Input: part model. Units: mm. Frame: model coordinates. Face numbers are marked on the shaded views. A direction names the side the tool comes from. Coordinates: 2 decimals unless noted, no trailing zeros. Order: outer loops, then holes, each group sorted by start corner. A loop starts at its lowest first (then second) coordinate and runs counter-clockwise, first axis right, second up.
Autodesk Inventor part; units mm, degrees
ref_plane "YZ Plane" through (0, 0, 0) normal (1, 0, 0) x (0, 1, 0)
ref_plane "XZ Plane" through (0, 0, 0) normal (0, 1, 0) x (-1, 0, 0)
ref_plane "XY Plane" through (0, 0, 0) normal (0, 0, 1) x (1, 0, 0)
sketch "草圖1" plane through (0, 0, 0) normal (0, 0, 1) x (1, 0, 0)
  line L0 (0, 0) -> (50, 0)
  line L1 (50, 10) -> (10, 10)
  line L2 (10, 10) -> (10, 40)
  line L3 (10, 40) -> (30, 40)
  line L4 (30, 40) -> (30, 50)
  line L5 (30, 50) -> (0, 50)
  line L6 (0, 50) -> (0, 0)
  line L7 (50, 10) -> (50, 0)
  dimension "d0" = 50
  dimension "d1" = 10
  dimension "d2" = 30
  dimension "d3" = 30
  dimension "d4" = 10
  dimension "d5" = 50
extrude "擠出1" add sketch "草圖1" along normal mid plane 40
fillet "圓角1" radius 20 2 edges at (50, 5, 20) (50, 5, -20)
fillet "圓角2" radius 20 1 edges at (0, 0, 0)
fillet "圓角3" radius 10 1 edges at (10, 10, 0)
fillet "圓角4" radius 10 2 edges at (30, 45, 20) (30, 45, -20)
sketch "草圖2" plane through (30, 10, 0) normal (0, 1, 0) x (1, 0, 0)
  arc A0 (0, -20) -> (0, 20) centre (0, 0) ccw
  point P0 (-30, 0)
hole "孔1" at (30, 10, 0) direction (0, -1, 0) diameter 20 end through all
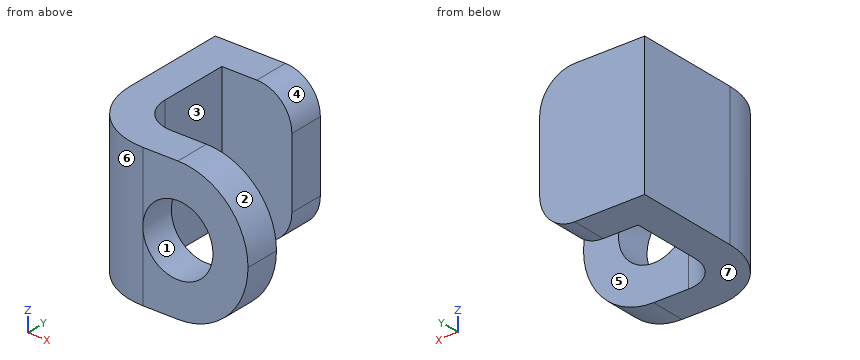
Item 1: Pin query (flat end, axial travel): pin 1 Ø16 at (y, z) = (31, -2) entering from +X; pin 2 Ø6 at (y, z) = (9.5, -3.5) entering from +X; pin 3 Ø10 at (y, z) = (43, 12.5) entering from +X; pin 4 Ø12 at (x, y) = (34.5, 33.5) entering from +Z. Return the tip coordinate at first contact, or that it passes through.
Response values:
pin 1: stops at x = 10
pin 2: stops at x = 49.99
pin 3: stops at x = 30
pin 4: passes through
Item 2: Cut plane B-B on x = 37. Return loops of the section in (y, z), then the cut area to 3 significant figures.
Response values:
outline: (0, -18.74) - (10, -18.74) - (10, -7.14) - (0, -7.14) - close; (0, 7.14) - (10, 7.14) - (10, 18.74) - (0, 18.74) - close
area: 232 mm2
Item 3: Draft query along Y for the marked faces 5, 6 and 7. Return one class per face: pulls with the +Y half, pulls with the -Y half, needs draft (parallel to the pull), parting line crosses it, or undercut.
Response values:
face 5: undercut
face 6: pulls with the -Y half
face 7: needs draft
Item 4: Ray query, probe 1 along Z at (x, y) = (30, 2); probe 2 along Y at (x, z) = (20, 16.5); probe 3 along Y at (x, z) = (41.5, 2). Return the intervals inside material, ascending.
Response values:
probe 1: z = -20 to -10, 10 to 20
probe 2: y = 0 to 10, 40 to 50
probe 3: y = 0 to 10
Item 5: Access query for the marked faces 1, 2, 3 and 4. Directions: +Z, -Z, +X, -X, +Y, -Y. A direction counts if a zero-diameter tool reaches every point of the face in a straight line with its end or side. Return the directions, or none.
Response values:
face 1: -Y
face 2: +Z, +X, +Y, -Y
face 3: +Z, -Z, +X
face 4: +Z, +X, +Y
Item 6: Cut plane A-A on z = -3. Return loops of the section in (x, y), then the cut area to 3 significant figures.
Response values:
outline: (0, 20) arc R20 ccw to (20, 0) - (20.46, 0) - (20.46, 10) - (20, 10) arc R10 cw to (10, 20) - (10, 40) - (30, 40) - (30, 50) - (0, 50) - close; (39.54, 0) - (49.77, 0) - (49.77, 10) - (39.54, 10) - close
area: 843 mm2
Item 7: Cut plane C-C on y = 41.5. Return loops of the section in (x, z), then the cut area to 3 significant figures.
Response values:
outline: (0, -20) - (20, -20) arc R10 ccw to (30, -10) - (30, 10) arc R10 ccw to (20, 20) - (0, 20) - close
area: 1,160 mm2
